For this review, take the finished solid that the model builds, in its own axes (mm). A direction names the side the tool comes from. Coordinates: 2 decimals unless noted, no trailing zeros. Loops run counter-clockwise (first coordinate to the right, second up) from the corner with the lowest first, then second, coordinate; pieces in that order, holes last. Notation, with made-up numbers: (29.25, 21.25) -> (75.25, 21.25) arc R32 ccw to (75.25, 58.25) -> close; hole circle Ø9 at (53, 79). An arc over 180 degrees is marked (long way). Answer in a Markdown table with one row per item.
Autodesk Inventor part; units mm, degrees
ref_plane "РабПлоскость1" through (-81.2124, 0, 0) normal (0, -1, 0) x (1, 0, 0)
ref_plane "YZ Plane" through (0, 0, 0) normal (1, 0, 0) x (0, 1, 0)
ref_plane "XZ Plane" through (0, 0, 0) normal (0, 1, 0) x (-1, 0, 0)
sketch "Эскиз1" plane through (0, 0, 0) normal (0, 0, 1) x (1, 0, 0)
  line L0 (-100, -75) -> (100, -75)
  line L1 (100, -75) -> (100, 75)
  line L2 (100, 75) -> (-100, 75)
  line L3 (-100, 75) -> (-100, -75)
  line L4 (-100, -75) -> (100, 75) construction
  line L5 (100, -75) -> (-100, 75) construction
  point P0 (0, 0)
  dimension "d0" = 200
  dimension "d1" = 150
extrude "Выдавливание1" add sketch "Эскиз1" along normal blind 5
sketch "Эскиз2" plane through (0, 0, 5) normal (0, 0, 1) x (1, 0, 0)
  line L0 (-100, -75) -> (100, -75)
  line L1 (100, -75) -> (100, 75)
  line L2 (100, 75) -> (-100, 75)
  line L3 (-100, 75) -> (-100, -75)
  line L4 (100, 75) -> (-100, 75) construction
  line L5 (0, 75) -> (0, -75) construction
  line L6 (-100, 0) -> (100, 0) construction
  line L7 (100, -75) -> (100, 75) construction
  line L8 (-100, -12.5) -> (100, -12.5) construction
  line L9 (100, -12.5) -> (100, 12.5) construction
  line L10 (100, 12.5) -> (-100, 12.5) construction
  line L11 (-100, 12.5) -> (-100, -12.5) construction
  line L12 (-100, -12.5) -> (100, 12.5) construction
  line L13 (100, -12.5) -> (-100, 12.5) construction
  line L14 (-100, 0) -> (0, 0) construction
  line L15 (-51.2124, 75) -> (-51.2124, -75) construction
  line L16 (-100, -75) -> (100, -75) construction
  line L17 (0, 0) -> (100, 0) construction
  line L18 (50, 75) -> (50, -75) construction
  line L19 (-81.2124, -12.5) -> (-21.2124, -12.5)
  line L20 (-21.2124, -12.5) -> (-21.2124, 12.5)
  line L21 (-21.2124, 12.5) -> (-81.2124, 12.5)
  line L22 (-81.2124, 12.5) -> (-81.2124, -12.5)
  line L23 (-81.2124, -12.5) -> (-21.2124, 12.5) construction
  line L24 (-21.2124, -12.5) -> (-81.2124, 12.5) construction
  line L25 (81.2124, -12.5) -> (21.2124, -12.5)
  line L26 (21.2124, -12.5) -> (21.2124, 12.5)
  line L27 (21.2124, 12.5) -> (81.2124, 12.5)
  line L28 (81.2124, 12.5) -> (81.2124, -12.5)
  point P0 (-51.2124, 0)
  dimension "d4" = 25
  dimension "d5" = 60
extrude "Выдавливание2" cut sketch "Эскиз2" against normal blind 5 contours L22 L21 L20 L19 | L25 L26 L27 L28
sketch "Эскиз3" plane through (-81.2124, 12.5, 5) normal (0, -1, 0) x (1, 0, 0)
  line L0 (0, 0) -> (60, 0)
  line L1 (30, 0) -> (30, 14.9537) construction
  line L2 (30, 0) -> (40, 0) construction
  line L3 (30, 0) -> (35, 0) construction
  line L4 (30, 0) -> (25, 0) construction
  line L5 (25, 0) -> (35, 0) construction
  line L6 (25, 0) -> (35, 0)
  line L7 (30, 0) -> (30, 3) construction
  circle A0 centre (30, 1.5) radius 1.5
  arc A1 (32.3946, 0.7816) -> (27.6054, 0.7816) centre (30, 1.5) ccw
  line L8 (35, 0) -> (32.3946, 0.7816)
  line L9 (25, 0) -> (27.6054, 0.7816)
  point P0 (81.2124, -5)
  dimension "d8" = 10
  dimension "d9" = 5
  dimension "d10" = 5
  dimension "d11" = 3
  dimension "d12" = 1
extrude "Выдавливание3" add sketch "Эскиз3" against normal blind 5
mirror "Зеркальное отражение1" about plane through (0, 0, 0) normal (0, 1, 0) of "Выдавливание3"
sketch "Эскиз4" plane through (-81.2124, 12.5, 0) normal (0, -1, 0) x (1, 0, 0)
  circle A0 centre (30, 6.5) radius 1.5
  point P0 (81.2124, 0)
surface extrude "ВыдавПврх1" sketch "Эскиз4" along normal up to next shown yes curves A0
boundary_patch "Участок поверхности1"
boundary_patch "Участок поверхности2"
ref_plane "РабПлоскость1" through (-81.2124, 0, 0) normal (0, -1, 0) x (1, 0, 0)
sketch "Эскиз6" plane through (0, 0, 5) normal (0, 0, 1) x (1, 0, 0)
  line L0 (81.2124, -12.5) -> (21.2124, -12.5)
  line L1 (21.2124, -12.5) -> (21.2124, 12.5)
  line L2 (21.2124, 12.5) -> (81.2124, 12.5)
  line L3 (81.2124, 12.5) -> (81.2124, -12.5)
  line L4 (-100, -75) -> (100, -75)
  line L5 (100, -75) -> (100, 75)
  line L6 (100, 75) -> (-100, 75)
  line L7 (-100, 75) -> (-100, -75)
  line L8 (-46.2124, -12.5) -> (-46.2124, -17.5)
  line L9 (-46.2124, -17.5) -> (-51.2124, -17.5)
  line L10 (-51.2124, -17.5) -> (-56.2124, -17.5)
  line L11 (-56.2124, -17.5) -> (-56.2124, -12.5)
  line L12 (-56.2124, -12.5) -> (-81.2124, -12.5)
  line L13 (-81.2124, -12.5) -> (-81.2124, 12.5)
  line L14 (-81.2124, 12.5) -> (-56.2124, 12.5)
  line L15 (-56.2124, 12.5) -> (-56.2124, 17.5)
  line L16 (-56.2124, 17.5) -> (-51.2124, 17.5)
  line L17 (-51.2124, 17.5) -> (-46.2124, 17.5)
  line L18 (-46.2124, 17.5) -> (-46.2124, 12.5)
  line L19 (-46.2124, 12.5) -> (-21.2124, 12.5)
  line L20 (-21.2124, 12.5) -> (-21.2124, -12.5)
  line L21 (-21.2124, -12.5) -> (-46.2124, -12.5)
  line L22 (-100, -75) -> (100, -75) construction
  line L23 (-21.2124, -75) -> (-21.2124, 75) construction
  line L24 (100, 75) -> (-100, 75) construction
  line L25 (-21.2124, 12.5) -> (-21.2124, 75) construction
  line L26 (-21.2124, 75) -> (21.2124, 75) construction
  line L27 (21.2124, 75) -> (21.2124, 12.5) construction
  line L28 (21.2124, 12.5) -> (-21.2124, 12.5) construction
  line L29 (-21.2124, 12.5) -> (-21.2124, 75) construction
  line L30 (-21.2124, -75) -> (21.2124, -75) construction
  line L31 (21.2124, -75) -> (21.2124, -12.5) construction
  line L32 (21.2124, -12.5) -> (-21.2124, -12.5) construction
  line L33 (-21.2124, -12.5) -> (-21.2124, -75) construction
  line L34 (100, -75) -> (100, 75) construction
  line L35 (-100, -7.5) -> (100, -7.5) construction
  line L36 (100, -7.5) -> (100, 7.5) construction
  line L37 (100, 7.5) -> (-100, 7.5) construction
  line L38 (-100, 7.5) -> (-100, -7.5) construction
  line L39 (-100, -7.5) -> (100, 7.5) construction
  line L40 (100, -7.5) -> (-100, 7.5) construction
  line L41 (0, 7.5) -> (0, 17.5) construction
  line L42 (0, -7.5) -> (0, -28.0993) construction
  line L43 (-2.5, -7.5) -> (-2.5, -28.0993)
  line L44 (2.5, -28.0993) -> (2.5, -7.5)
  arc A0 (2.5, -7.5) -> (-2.5, -7.5) centre (0, -7.5) ccw
  line L45 (-2.5, -28.0993) -> (-2.5, -38.0993)
  line L46 (2.5, -28.0993) -> (2.5, -38.0993)
  arc A1 (-2.5, -38.0993) -> (2.5, -38.0993) centre (0, -38.0993) ccw
  line L47 (-21.2124, 0) -> (21.2124, 0) construction
  line L48 (-2.5, 7.5) -> (-2.5, 28.0993)
  line L49 (2.5, 28.0993) -> (2.5, 7.5)
  arc A2 (-2.5, 7.5) -> (2.5, 7.5) centre (0, 7.5) ccw
  line L50 (-2.5, 28.0993) -> (-2.5, 38.0993)
  line L51 (2.5, 28.0993) -> (2.5, 38.0993)
  arc A3 (2.5, 38.0993) -> (-2.5, 38.0993) centre (0, 38.0993) ccw
  point P0 (0, 0)
  point P1 (0, -17.7997)
  point P2 (0, 17.7997)
  dimension "d24" = 15
  dimension "d25" = 10
  dimension "d27" = 10
extrude "Выдавливание5" cut sketch "Эскиз6" against normal blind 20 contours A0 L44 L46 A1 L45 L43 | L48 L50 A3 L51 L49 A2
mirror "Зеркальное отражение2" about plane through (0, 0, 0) normal (1, 0, 0) of "Выдавливание3", "ВыдавПврх1", "Зеркальное отражение1"
sketch "Эскиз7" plane through (0, 0, 5) normal (0, 0, 1) x (1, 0, 0)
  arc A0 (-2.5, -38.0993) -> (2.5, -38.0993) centre (0, -38.0993) ccw
  line L0 (-2.5, -38.0993) -> (-2.5, -7.5)
  arc A1 (2.5, -7.5) -> (-2.5, -7.5) centre (0, -7.5) ccw
  line L1 (2.5, -7.5) -> (2.5, -38.0993)
  arc A2 (2.5, 38.0993) -> (-2.5, 38.0993) centre (0, 38.0993) ccw
  line L2 (2.5, 38.0993) -> (2.5, 7.5)
  arc A3 (-2.5, 7.5) -> (2.5, 7.5) centre (0, 7.5) ccw
  line L3 (-2.5, 7.5) -> (-2.5, 38.0993)
  line L4 (-100, -75) -> (100, -75)
  line L5 (100, -75) -> (100, 75)
  line L6 (100, 75) -> (-100, 75)
  line L7 (-100, 75) -> (-100, -75)
  line L8 (-46.2124, -12.5) -> (-46.2124, -17.5)
  line L9 (-46.2124, -17.5) -> (-51.2124, -17.5)
  line L10 (-51.2124, -17.5) -> (-56.2124, -17.5)
  line L11 (-56.2124, -17.5) -> (-56.2124, -12.5)
  line L12 (-56.2124, -12.5) -> (-81.2124, -12.5)
  line L13 (-81.2124, -12.5) -> (-81.2124, 12.5)
  line L14 (-81.2124, 12.5) -> (-56.2124, 12.5)
  line L15 (-56.2124, 12.5) -> (-56.2124, 17.5)
  line L16 (-56.2124, 17.5) -> (-51.2124, 17.5)
  line L17 (-51.2124, 17.5) -> (-46.2124, 17.5)
  line L18 (-46.2124, 17.5) -> (-46.2124, 12.5)
  line L19 (-46.2124, 12.5) -> (-21.2124, 12.5)
  line L20 (-21.2124, 12.5) -> (-21.2124, -12.5)
  line L21 (-21.2124, -12.5) -> (-46.2124, -12.5)
  line L22 (56.2124, -12.5) -> (56.2124, -17.5)
  line L23 (56.2124, -17.5) -> (51.2124, -17.5)
  line L24 (51.2124, -17.5) -> (46.2124, -17.5)
  line L25 (46.2124, -17.5) -> (46.2124, -12.5)
  line L26 (46.2124, -12.5) -> (21.2124, -12.5)
  line L27 (21.2124, -12.5) -> (21.2124, 12.5)
  line L28 (21.2124, 12.5) -> (46.2124, 12.5)
  line L29 (46.2124, 12.5) -> (46.2124, 17.5)
  line L30 (46.2124, 17.5) -> (51.2124, 17.5)
  line L31 (51.2124, 17.5) -> (56.2124, 17.5)
  line L32 (56.2124, 17.5) -> (56.2124, 12.5)
  line L33 (56.2124, 12.5) -> (81.2124, 12.5)
  line L34 (81.2124, 12.5) -> (81.2124, -12.5)
  line L35 (81.2124, -12.5) -> (56.2124, -12.5)
  line L36 (-100, 75) -> (-70, 75) construction
  line L37 (-70, 75) -> (-70, 45) construction
  line L38 (-70, 45) -> (-100, 45) construction
  line L39 (-100, 45) -> (-100, 75) construction
  circle A4 centre (-70, 45) radius 2.5
  line L40 (100, -75) -> (100, 75) construction
  line L41 (100, 0) -> (-100, 0) construction
  line L42 (100, 75) -> (-100, 75) construction
  line L43 (0, 75) -> (0, -75) construction
  line L44 (-100, -75) -> (100, -75) construction
  circle A5 centre (70, 45) radius 2.5
  line L45 (-100, -75) -> (100, -75)
  line L46 (-70, -75) -> (-70, -35) construction
  line L47 (-70, -35) -> (-100, -35) construction
  circle A6 centre (-70, -35) radius 2.5
  line L48 (70, -75) -> (70, -35) construction
  line L49 (70, -35) -> (100, -35) construction
  circle A7 centre (70, -35) radius 2.5
  line L50 (-100, -75) -> (-100, -55)
  line L51 (-100, -55) -> (100, -55)
  line L52 (100, -75) -> (100, -55)
  point P0 (0, 0)
  dimension "d30" = 30
  dimension "d31" = 30
  dimension "d32" = 5
  dimension "d35" = 40
  dimension "d36" = 5
  dimension "d37" = 20
extrude "Выдавливание6" cut sketch "Эскиз7" against normal blind 20 contours L7 L51 L5 L4 | A4 | A5 | A6 | A7
properties part number "Down"
Item 1: For L1, parallel to X at y = 14.1, z = 6.5; L2, parallel to Y at x = 70, z = 2.2; L3, parallel to X at y = -20, z = 2.5, list the stretches that pass through material, from the lowest coordinate up.
Worked answers:
| item | result |
|---|---|
| L1 | -53.71 to -52.71, -49.71 to -48.71, 48.71 to 49.71, 52.71 to 53.71 |
| L2 | -55 to -37.5, -32.5 to -12.5, 12.5 to 42.5, 47.5 to 75 |
| L3 | -100 to -2.5, 2.5 to 100 |
Item 2: Take a section at C-C, the plane y = 23. State the section outline as (x, z) points.
Worked answers:
| item | result |
|---|---|
| outline | (-100, 0) -> (-2.5, 0) -> (-2.5, 5) -> (-100, 5) -> close; (2.5, 0) -> (100, 0) -> (100, 5) -> (2.5, 5) -> close |
Item 3: The part is to be moulded in two halves that separate along Z. For faces 4 (the cylindrical face through (-51.15, 14.96, 9)), 5 (the flat face through (1, 75, 2)), 6 (the flat face through (-1, -4, 5)), say which applies: +Z half, -Z half, draft (parallel to the pull), parting line (faces both ways), or undercut.
Worked answers:
| item | result |
|---|---|
| face 4 | undercut |
| face 5 | draft |
| face 6 | +Z half |
Item 4: Take a section at B-B, the plane x = -70. State the section outline as (y, z) points, and give its area (3 significant figures).
Worked answers:
| item | result |
|---|---|
| outline | (-55, 0) -> (-37.5, 0) -> (-37.5, 5) -> (-55, 5) -> close; (-32.5, 0) -> (-12.5, 0) -> (-12.5, 5) -> (-32.5, 5) -> close; (12.5, 0) -> (42.5, 0) -> (42.5, 5) -> (12.5, 5) -> close; (47.5, 0) -> (75, 0) -> (75, 5) -> (47.5, 5) -> close |
| area | 475 mm² |
Item 5: For faces 1 (the cylindrical face through (0, -5, 3)), 2 (the flat face through (52, -17.5, 8)), 3 (the flat face through (-52, 17.5, 8)), list the 3-axis set-ups (+Z, -Z, +X, -X, +Y, -Y) from which the entire face can be reached by the end or side of a thin tool; tool diameter is ignored.
Worked answers:
| item | result |
|---|---|
| face 1 | +Z, -Z |
| face 2 | +Z, +X, -X, -Y |
| face 3 | +Z, +X, -X, +Y |
Item 6: Take a section at D-D, the plane y = -1.5. State the section outline as (x, z) points, and give its area (3 significant figures).
Worked answers:
| item | result |
|---|---|
| outline | (-100, 0) -> (-81.21, 0) -> (-81.21, 5) -> (-100, 5) -> close; (-21.21, 0) -> (21.21, 0) -> (21.21, 5) -> (-21.21, 5) -> close; (81.21, 0) -> (100, 0) -> (100, 5) -> (81.21, 5) -> close |
| area | 400 mm² |
Item 7: Take a section at A-A, the plane y = -35. State the section outline as (x, z) points, and give its area (3 significant figures).
Worked answers:
| item | result |
|---|---|
| outline | (-100, 0) -> (-72.5, 0) -> (-72.5, 5) -> (-100, 5) -> close; (-67.5, 0) -> (-2.5, 0) -> (-2.5, 5) -> (-67.5, 5) -> close; (2.5, 0) -> (67.5, 0) -> (67.5, 5) -> (2.5, 5) -> close; (72.5, 0) -> (100, 0) -> (100, 5) -> (72.5, 5) -> close |
| area | 925 mm² |
Item 8: Insertion check: pin 1 (3 mm diameter, centred on x = 53.5, z = 7.5, fed in from -Y); pin 2 (4 mm diameter, centred on x = -41, y = 35, fed in from -Z); pin 3 (3 mm diameter, centred on x = 51, z = 7.5, fed in from +Y). Each pin has a flat end and moves straight along its axis. Give the tip position at first contact, or say it passes through.
Worked answers:
| item | result |
|---|---|
| pin 1 | y = -17.5 |
| pin 2 | z = 0 |
| pin 3 | y = 17.5 |
